Verification items for this drawing (mm, ordinates from the low corner). A direction names the side the tool comes from. Coordinates: 2 decimals unless noted, no trailing zeros. Loops run counter-clockwise (first coordinate to the right, second up) from the corner with the lowest first, then second, coordinate; pieces in that order, holes last. Notation, with made-up numbers: M 60,-25 L 67,-25 A23 ccw 67,-12 Z; hole C 3,29 d4. An arc over 180 degrees is marked long. Use CSV: the item, a comma, the result in double quotes.
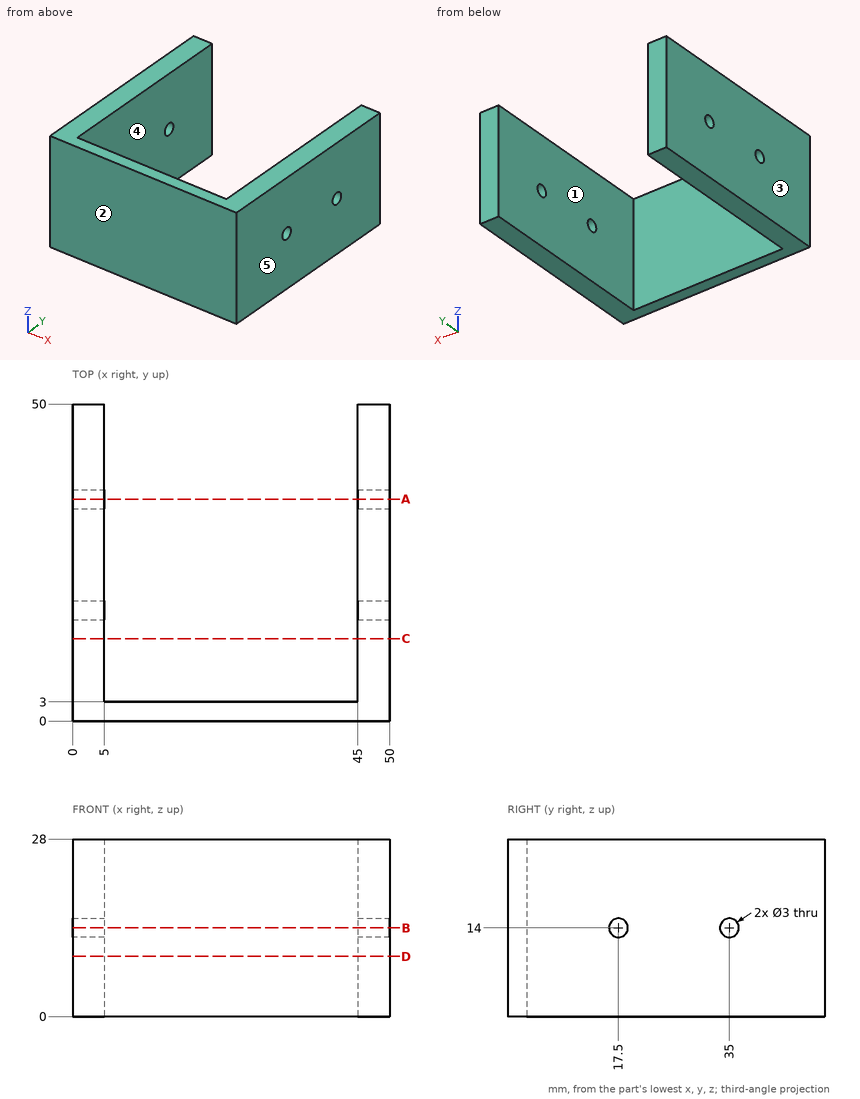
1. Release check for a two-part mould opening along X. For the marked faces 3, 4 and 5 record: +X half, -X half, draft (parallel to the pull), parting line (faces both ways), or undercut.
The answers:
face 3,"-X half"
face 4,"undercut"
face 5,"+X half"
2. Thickness scan on line 1 (Y direction, x = 1.2, z = 14); line 2 (X direction, y = 15.5, z = 22.25); line 3 (Y direction, x = 29, z = 11). Record the ranges inside material, lowest first. Write a range as [from, to].
The answers:
line 1,"[0, 16], [19, 33.5], [36.5, 50]"
line 2,"[0, 5], [45, 50]"
line 3,"[0, 3]"
3. Section check A-A, the plane y = 35. Record the cut outline in (x, z).
The answers:
outline,"M 0,0 L 5,0 L 5,12.5 L 0,12.5 Z; M 0,15.5 L 5,15.5 L 5,28 L 0,28 Z; M 45,0 L 50,0 L 50,12.5 L 45,12.5 Z; M 45,15.5 L 50,15.5 L 50,28 L 45,28 Z"
4. Gauge pin test, flat end, axial feed: P1, Ø3, axis at x = 42.5, y = 14.5, coming from the -Z side. Record the tip position at first contact, or that the pin passes through.
The answers:
P1,"through"
5. Section check B-B, the plane z = 14. Record the cut outline in (x, y).
The answers:
outline,"M 0,0 L 50,0 L 50,16 L 45,16 L 45,3 L 5,3 L 5,16 L 0,16 Z; M 0,19 L 5,19 L 5,33.5 L 0,33.5 Z; M 0,36.5 L 5,36.5 L 5,50 L 0,50 Z; M 45,19 L 50,19 L 50,33.5 L 45,33.5 Z; M 45,36.5 L 50,36.5 L 50,50 L 45,50 Z"
6. Set-up check for the marked faces 1 and 2: record each of +Z, -Z, +X, -X, +Y, -Y from which the full face is reachable in a straight line by a thin tool's end or side.
The answers:
face 1,"+Z, -Z, +Y"
face 2,"+Z, -Z, +X, -X, -Y"
7. Section check C-C, the plane y = 13. Record the cut outline in (x, z).
The answers:
outline,"M 0,0 L 5,0 L 5,28 L 0,28 Z; M 45,0 L 50,0 L 50,28 L 45,28 Z"
8. Section check D-D, the plane z = 9.5. Record the cut outline in (x, y), plus the area to 3 significant figures.
The answers:
outline,"M 0,0 L 50,0 L 50,50 L 45,50 L 45,3 L 5,3 L 5,50 L 0,50 Z"
area,"620 mm^2"
